Source: CAD feature listing. Evaluate the final solid. Frame: model axes, mm. A direction names the side the tool comes from. Coordinates: 2 decimals unless noted, no trailing zeros. Write each loop counter-clockwise with the first axis right and the second up, starting at its lowest first coordinate (ties: lowest second). Pieces come first, ordered by that corner, then holes. Notation, with made-up numbers: (79, -7) -> (136, -7) arc R35 ccw to (136, 27) -> close; hole circle Ø11 at (28, 81). An arc over 180 degrees is marked (long way). One line per item, written item: value. Start each with the question number.
1. Section query C-C, the plane z = 1. State how many separate pieces and enclosed holes the cut face has, and give its area (3 significant figures).
2. Section query B-B, the plane x = -17.5. Output: boundary loops of the cut face in (y, z), and give its area (3 significant figures).
3. Section query D-D, the plane y = -6.75. Output: boundary loops of the cut face in (x, z), and give its area (3 significant figures).
4. Line query: line 1 (Y direction, x = -16.5, z = -3); line 2 (Z direction, x = 0, y = -3.85); line 3 (Z direction, x = 17.5, y = -2.15). Output: solid intervals per line, ascending.
5. Mould query, pull axis X, two halves, no side actions, for faces 4 (the cylindrical face through (15.9, -1.48, -0.07)), 5 (the flat face through (-7, -8.4, -6)), 6 (the cylindrical face through (22.5, -1.5, 0.1)). Classes: released by +X, released by -X, zero draft, split by the parting line, or undercut.
6. Access query for faces 1 (the cylindrical face through (-2.222, -2.757, -10.006)), 2 (the cylindrical face through (-12.488, -5.075, -0.55)), 3 (the flat face through (-12.6, -1.48, 7.86)). Directions: +Z, -Z, +X, -X, +Y, -Y. A direction counts if a zero-diameter tool reaches every point of the face in a straight line with its end or side. Return the directions, or none.
7. First-contact query: P1, Ø1.5, axis at y = -7.5, z = 9, coming from the +X side; P2, Ø1.9, axis at x = 17.5, z = 0, coming from the +Y side; P3, Ø2, axis at x = 10, y = -7, coming from the +Z side; P4, Ø4, axis at x = 5.5, y = -1.5, coming from the -Z side. Flat tips, straight axial feed; report the tip coordinate or a pass-through.
8. Section query A-A, the plane y = -2. Output: boundary loops of the cut face in (x, z).
from build123d import *

# Parameters (mm, degrees)
SKETCH1_R               = 12.5
BOSS_EXTRUDE1_DEPTH     = 8.4
SKETCH2_R               = 10.25
CUT_EXTRUDE1_DEPTH      = 1
CUT_EXTRUDE1_DEPTH_BACK = 9.4
SKETCH4_R               = 1.6
BOSS_EXTRUDE2_DEPTH     = 3


with BuildPart() as part:
    # Sketch1 → Boss-Extrude1 (new body)
    with BuildSketch(Plane(origin=(0, 0, 0), x_dir=(1, 0, 0), z_dir=(0, 1, 0))):
        Circle(SKETCH1_R)
    extrude(amount=-BOSS_EXTRUDE1_DEPTH)

    # Sketch2 → Cut-Extrude1 (cut, two sides)
    with BuildSketch(Plane.XZ.offset(8.4)) as cut_extrude1_sk:
        Circle(SKETCH2_R)
    extrude(amount=CUT_EXTRUDE1_DEPTH, mode=Mode.SUBTRACT)
    extrude(cut_extrude1_sk.sketch, amount=-CUT_EXTRUDE1_DEPTH_BACK, mode=Mode.SUBTRACT)

    # Sketch3 → Revolve1 (revolve)
    with BuildSketch(Plane(origin=(0, 0, 0), x_dir=(0, 0, -1), z_dir=(1, 0, 0))):
        Polygon((9.023871751, -8.4), (12.5, 0), (12.5, -8.4), align=None)
    revolve(axis=Axis((0, -24.717, 0), (0, 1, 0)))

    # Sketch4 → Boss-Extrude2 (add)
    with BuildSketch(Plane(origin=(0, 0, 0), x_dir=(1, 0, 0), z_dir=(0, 1, 0))):
        with BuildLine():
            Line((-5.357142857, 11.293848786), (-19.642857143, 4.517539515))
            ThreePointArc((-19.642857143, 4.517539515), (-22.5, 0), (-19.642857143, -4.517539515))
            Line((-19.642857143, -4.517539515), (-5.357142857, -11.293848786))
            ThreePointArc((-5.357142857, -11.293848786), (-12.5, 0), (-5.357142857, 11.293848786))
        make_face()
        with Locations((-17.5, 0)):
            Circle(SKETCH4_R, mode=Mode.SUBTRACT)
        with BuildLine():
            Line((5.357142857, -11.293848786), (19.642857143, -4.517539515))
            ThreePointArc((19.642857143, -4.517539515), (22.5, 0), (19.642857143, 4.517539515))
            Line((19.642857143, 4.517539515), (5.357142857, 11.293848786))
            ThreePointArc((5.357142857, 11.293848786), (12.5, 0), (5.357142857, -11.293848786))
        make_face()
        with Locations((17.5, 0)):
            Circle(SKETCH4_R, mode=Mode.SUBTRACT)
    extrude(amount=-BOSS_EXTRUDE2_DEPTH)


solid = part.part
Computed values:
1. separate pieces: 4
1. enclosed holes: 0
1. area: 86.2 mm²
2. outline: (-3, -5.53) -> (0, -5.53) -> (0, -1.6) -> (-3, -1.6) -> close; (-3, 1.6) -> (0, 1.6) -> (0, 5.53) -> (-3, 5.53) -> close
2. area: 23.6 mm²
3. outline: circle Ø25 at (0, 0); hole circle Ø19.41 at (0, 0)
3. area: 195 mm²
4. line 1: y = -3 to 0
4. line 2: z = -12.5 to -10.25, 10.25 to 12.5
4. line 3: z = -5.53 to -1.6, 1.6 to 5.53
5. face 4: undercut
5. face 5: zero draft
5. face 6: released by +X
6. face 1: +Y
6. face 2: -Y
6. face 3: +Z, -X, +Y, -Y
7. P1: stops at x = 9.39
7. P2: passes through
7. P3: stops at z = 8.67
7. P4: stops at z = -12
8. outline: (-19.64, -4.52) -> (-5.36, -11.29) arc R12.5 ccw to (5.36, -11.29) -> (19.64, -4.52) arc R5 ccw to (19.64, 4.52) -> (5.36, 11.29) arc R12.5 ccw to (-5.36, 11.29) -> (-19.64, 4.52) arc R5 ccw to start; hole circle Ø3.2 at (-17.5, 0); hole circle Ø20.5 at (0, 0); hole circle Ø3.2 at (17.5, 0)
